Input: part model. Units: mm. Frame: model coordinates. A direction names the side the tool comes from. Coordinates: 2 decimals unless noted, no trailing zeros. Loops run counter-clockwise (first coordinate to the right, second up) from the corner with the lowest first, then second, coordinate; pieces in that order, holes last. Notation, with made-up numbers: (17, -36.75) - (51, -36.75) arc R14 cw to (51, -14.75) - close; hole circle Ø5 at (58.5, 4). An arc over 180 degrees is marked (long way). Use one line per item in the form item = value.
from build123d import *

# Parameters (mm, degrees)
SKETCH1_R      = 7
EXTRUDE1_DEPTH = 37
EXTRUDE3_START = -4
EXTRUDE3_DEPTH = 35.301436004
SKETCH4_R      = 7
SKETCH4_R_2    = 6
EXTRUDE4_DEPTH = 10
CHAMFER1_SIZE  = 0.5


with BuildPart() as part:
    # Sketch1 → Extrude1 (new, symmetric)
    with BuildSketch(Plane.XY):
        Circle(SKETCH1_R)
    extrude(amount=EXTRUDE1_DEPTH, both=True)

    # Sketch3 → Extrude3 (cut, through all)
    with BuildSketch(Plane(origin=(0, 0, 0), x_dir=(1, 0, 0), z_dir=(0, 1, 0)).offset(EXTRUDE3_START)):
        with BuildLine():
            Line((-2.5, -27), (-2.5, 27))
            ThreePointArc((-2.5, 27), (0, 29.5), (2.5, 27))
            Line((2.5, 27), (2.5, -27))
            ThreePointArc((2.5, -27), (0, -29.5), (-2.5, -27))
        make_face()
    extrude(amount=-EXTRUDE3_DEPTH, mode=Mode.SUBTRACT)

    # Sketch4 → Extrude4 (cut)
    with BuildSketch(Plane.XY.offset(37)):
        with Locations(Location((0, 0, 0), (0, 0, 249.075167572))):
            Circle(SKETCH4_R)
        Circle(SKETCH4_R_2, mode=Mode.SUBTRACT)
    extrude4 = extrude(amount=-EXTRUDE4_DEPTH, mode=Mode.SUBTRACT)

    # Mirror1: Extrude4 across plane
    add(extrude4.mirror(Plane.XY), mode=Mode.SUBTRACT)

    # Chamfer1
    chamfer1_edges = [part.edges().sort_by_distance(p)[0] for p in [
        (0, 7, 27),
        (-6, 0, 37),
        (0, 7, -27),
        (-6, 0, -37),
    ]]
    chamfer(chamfer1_edges, length=CHAMFER1_SIZE)


solid = part.part
Q1. First-contact query: P1, Ø3, axis at y = -5.5, z = 4, coming from the +X side; P2, Ø2.5, axis at x = -0.5, z = -5.5, coming from the -Y side; P3, Ø6, axis at y = 5.5, z = -21.5, coming from the -X side. Flat tips, straight axial feed; report the tip coordinate or a pass-through.
Check values:
P1 = 5.74
P2 = -4
P3 = -6.54
Q2. Set-up query: faces 1 (the flat face through (-2, 6, 27)), 2 (the flat face through (-2.5, -5, 0)), 3 (the flat face through (0, 0, -37)), 4 (the cylindrical face through (0, 7, 0)), 5 (the cylindrical face through (-0.78, 5.95, -31.82)). Return all of +Z, -Z, +X, -X, +Y, -Y with unobstructed straight access to the full face (end or side cutting, diameter ignored); none if empty.
Check values:
face_1 = +Z
face_2 = -Y
face_3 = -Z, +X, -X, +Y, -Y
face_4 = +Z, -Z
face_5 = -Z
Q3. Cut plane D-D, the plane z = -5. Return loops of the section in (x, y), then the cut area to 3 significant figures.
Check values:
outline = (-2.5, -6.54) - (-2.5, -4) - (2.5, -4) - (2.5, -6.54) arc R7 ccw (long way) to start
area = 140 mm²
Q4. Cut plane A-A, the plane x = 0. Return loops of the section in (y, z).
Check values:
outline = (-6, -36.5) - (-5.5, -37) - (5.5, -37) - (6, -36.5) - (6, -27) - (6.5, -27) - (7, -26.5) - (7, 26.5) - (6.5, 27) - (6, 27) - (6, 36.5) - (5.5, 37) - (-5.5, 37) - (-6, 36.5) - (-6, 29.5) - (-4, 29.5) - (-4, -29.5) - (-6, -29.5) - close
Q5. Ray query, line 1 along X through (y, z) = (-4.75, -1.5); line 2 along Z through (x, y) = (-5, -3.5); line 3 along Z through (x, y) = (5.5, -2.25). Return the intervals inside material, ascending. Write a range as [from, to].
Check values:
line_1 = [-5.14, -2.5], [2.5, 5.14]
line_2 = [-27, 27]
line_3 = [-36.56, 36.56]
Q6. Cut plane C-C, the plane z = -31. Return loops of the section in (x, y).
Check values:
outline = circle Ø12 at (0, 0)
Q7. Cut plane B-B, the plane y = 0. Return loops of the section in (x, z), then the cut area to 3 significant figures.
Check values:
outline = (-7, -26.5) - (-6.5, -27) - (-6, -27) - (-6, -36.5) - (-5.5, -37) - (5.5, -37) - (6, -36.5) - (6, -27) - (6.5, -27) - (7, -26.5) - (7, 26.5) - (6.5, 27) - (6, 27) - (6, 36.5) - (5.5, 37) - (-5.5, 37) - (-6, 36.5) - (-6, 27) - (-6.5, 27) - (-7, 26.5) - close
area = 995 mm²
Q8. Pull-direction query (Z, two-part tool) for faces 6 (the cylindrical face through (-0.1, -4.8, -29.5)), 7 (the cylindrical face through (-0.78, 5.95, 31.82)), 8 (the flat face through (-2, 6, -27)); classes: pulls with the +Z half, pulls with the -Z half, needs draft (parallel to the pull), parting line crosses it, or undercut.
Check values:
face_6 = undercut
face_7 = needs draft
face_8 = pulls with the -Z half
